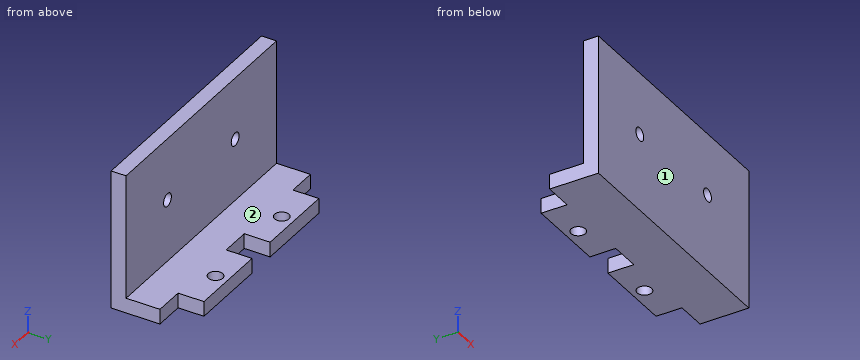
```python
from build123d import *

# Parameters (mm, degrees)
SKETCH1_W           = 50
SKETCH1_H           = 28
BOSS_EXTRUDE1_DEPTH = 3
SKETCH2_W           = 50
SKETCH2_H           = 3
BOSS_EXTRUDE2_DEPTH = 12
SKETCH6_W           = 6
SKETCH6_H           = 5.2
CUT_EXTRUDE2_DEPTH  = 3
SKETCH7_R           = 1.3
CUT_EXTRUDE3_DEPTH  = 3
SKETCH8_R           = 1.45
CUT_EXTRUDE4_DEPTH  = 3


with BuildPart() as part:
    # Sketch1 → Boss-Extrude1 (new body)
    with BuildSketch(Plane(origin=(0, 0, 0), x_dir=(1, 0, 0), z_dir=(0, 1, 0))):
        Rectangle(SKETCH1_W, SKETCH1_H)
    extrude(amount=BOSS_EXTRUDE1_DEPTH)

    # Sketch2 → Boss-Extrude2 (add)
    with BuildSketch(Plane(origin=(0, 3, 0), x_dir=(1, 0, 0), z_dir=(0, 1, 0))):
        with Locations((0, 12.5)):
            Rectangle(SKETCH2_W, SKETCH2_H)
    extrude(amount=BOSS_EXTRUDE2_DEPTH)

    # Sketch6 → Cut-Extrude2 (cut)
    with BuildSketch(Plane(origin=(0, 0, -14), x_dir=(-1, 0, 0), z_dir=(0, 0, -1))):
        with Locations((-22, 12.4)):
            Rectangle(SKETCH6_W, SKETCH6_H)
        with Locations((0, 12.4)):
            Rectangle(SKETCH6_W, SKETCH6_H)
        with Locations((22.191038301, 12.4)):
            Rectangle(SKETCH6_W, SKETCH6_H)
    extrude(amount=-CUT_EXTRUDE2_DEPTH, mode=Mode.SUBTRACT)

    # Sketch7 → Cut-Extrude3 (cut)
    with BuildSketch(Plane.XZ):
        with Locations((-11.25, 1.5)):
            Circle(SKETCH7_R)
        with Locations((11.25, 1.5)):
            Circle(SKETCH7_R)
    extrude(amount=-CUT_EXTRUDE3_DEPTH, mode=Mode.SUBTRACT)

    # Sketch8 → Cut-Extrude4 (cut)
    with BuildSketch(Plane(origin=(0, 0, -14), x_dir=(-1, 0, 0), z_dir=(0, 0, -1))):
        with Locations((-11, 12.5)):
            Circle(SKETCH8_R)
        with Locations((11, 12.5)):
            Circle(SKETCH8_R)
    extrude(amount=-CUT_EXTRUDE4_DEPTH, mode=Mode.SUBTRACT)


solid = part.part
```
Design review of the part built by this model. Coordinates are the model's own, in mm. Face numbers are marked on the shaded views. A direction names the side the tool comes from. Coordinates: 2 decimals unless noted, no trailing zeros. Order: outer loops, then holes, each group sorted by start corner. A loop starts at its lowest first (then second) coordinate and runs counter-clockwise, first axis right, second up. Notation, with made-up numbers: (-20.75, -15) -> (12.25, -15) arc R24 cw to (12.25, 18) -> close; hole circle Ø6 at (-7, -8.5). An arc over 180 degrees is marked (long way). One line per item, written item: value. Start each with the question number.
Q1. Take a section at C-C, the plane z = 1.5. State the section outline as (x, y) points.
Q2. Take a section at A-A, the plane x = 11.25. State the section outline as (y, z) points.
Q3. For probe 1 along Z at (x, y) = (-11.25, 1.1); probe 2 along Y at (x, z) = (16, 10.25); probe 3 along Z at (x, y) = (17, 4.25), list the stretches that pass through material, from the lowest coordinate up.
Q4. Insertion check: pin 1 Ø1.5 at (y, z) = (12.5, -13) entering from -X; pin 2 Ø0.9 at (y, z) = (13.5, -12.5) entering from +X; pin 3 Ø7.5 at (x, z) = (10, -0.5) entering from +Y; pin 4 Ø1.6 at (x, z) = (11.25, 1.5) entering from -Y. Each pin has a flat end and moves straight along its axis. Give the tip position at first contact, or say it passes through.
Q5. Take a section at B-B, the plane y = 13.25. State the section outline as (x, z) points, then the cut area to 3 significant figures.
Q6. Tool access review of the marked faces 1 and 2: name each direction out of +Z, -Z, +X, -X, +Y, -Y from which nothing blocks a thin tool from reaching the whole face with its end or side.
Q7. Take a section at D-D, the plane x = -1. State the section outline as (y, z) points.
Values follow:
1. outline: (-25, 0) -> (-12.55, 0) -> (-12.55, 3) -> (-25, 3) -> close; (-9.95, 0) -> (9.95, 0) -> (9.95, 3) -> (-9.95, 3) -> close; (12.55, 0) -> (25, 0) -> (25, 3) -> (12.55, 3) -> close
2. outline: (0, -14) -> (11.07, -14) -> (11.07, -11) -> (3, -11) -> (3, 0.2) -> (0, 0.2) -> close; (0, 2.8) -> (3, 2.8) -> (3, 14) -> (0, 14) -> close; (13.93, -14) -> (15, -14) -> (15, -11) -> (13.93, -11) -> close
3. probe 1: z = -14 to 0.2, 2.8 to 14
3. probe 2: y = 0 to 3
3. probe 3: z = -14 to -11
4. pin 1: stops at x = -19.19
4. pin 2: stops at x = 19
4. pin 3: stops at y = 3
4. pin 4: passes through
5. outline: (-19.19, -14) -> (-12.24, -14) -> (-12.24, -11) -> (-19.19, -11) -> close; (-9.76, -14) -> (-3, -14) -> (-3, -11) -> (-9.76, -11) -> close; (3, -14) -> (9.76, -14) -> (9.76, -11) -> (3, -11) -> close; (12.24, -14) -> (19, -14) -> (19, -11) -> (12.24, -11) -> close
5. area: 81.7 mm2
6. face 1: +Z, -Z, +X, -X, -Y
6. face 2: +Z, +X, -X, +Y
7. outline: (0, -14) -> (9.8, -14) -> (9.8, -11) -> (3, -11) -> (3, 14) -> (0, 14) -> close
